```python
from build123d import *

# Parameters (mm, degrees)
ESQUISSE1_W                  = 150
ESQUISSE1_H                  = 150
BOSS_EXTRU_1_DEPTH           = 3
ESQUISSE3_W                  = 130
ESQUISSE3_H                  = 10
ENL_V_MAT_EXTRU_1_DEPTH      = 3
ENL_V_MAT_EXTRU_2_DEPTH      = 153
ENL_V_MAT_EXTRU_2_DEPTH_BACK = 200
ESQUISSE4_R                  = 0.75
CONG_1_R                     = 1
BOSS_EXTRU_5_DEPTH           = 3
BOSS_EXTRU_6_DEPTH           = 3
CONG_4_R                     = 20


with BuildPart() as part:
    # Esquisse1 → Boss.-Extru.1 (new body)
    with BuildSketch(Plane.XY):
        with Locations((75, 75)):
            Rectangle(ESQUISSE1_W, ESQUISSE1_H)
    extrude(amount=BOSS_EXTRU_1_DEPTH)

    # Esquisse3 → Enlèv. mat.-Extru.1 (cut)
    with BuildSketch(Plane.XY.offset(3)):
        with Locations((75, 145)):
            Rectangle(ESQUISSE3_W, ESQUISSE3_H)
    extrude(amount=-ENL_V_MAT_EXTRU_1_DEPTH, mode=Mode.SUBTRACT)

    # Esquisse4 → Enlèv. mat.-Extru.2 (cut, two sides: drawn at the far end of the back side and taken through both)
    with BuildSketch(Plane(origin=(10, 0, 0), x_dir=(0, 0, -1), z_dir=(1, 0, 0)).offset(-ENL_V_MAT_EXTRU_2_DEPTH_BACK)):
        with Locations(Location((-1.5, 148, 0), (0, 0, 270))):
            Circle(ESQUISSE4_R)
    extrude(amount=ENL_V_MAT_EXTRU_2_DEPTH + ENL_V_MAT_EXTRU_2_DEPTH_BACK, mode=Mode.SUBTRACT)

    # Congé1
    cong_1_edges = [part.edges().sort_by_distance(p)[0] for p in [
        (145, 150, 3),
        (5, 150, 0),
        (5, 150, 3),
        (145, 150, 0),
    ]]
    fillet(cong_1_edges, radius=CONG_1_R)

    # Esquisse8 → Boss.-Extru.5 (add)
    with BuildSketch(Plane(origin=(150, 0, 0), x_dir=(0, 0, -1), z_dir=(1, 0, 0))):
        Polygon((0, 3), (68.936542711, -9.155372437), (59.757502948, 47.611044498), (0, 53), align=None)
    extrude(amount=-BOSS_EXTRU_5_DEPTH)

    # Esquisse9 → Boss.-Extru.6 (add)
    with BuildSketch(Plane.ZY):
        Polygon((0, 53), (-59.757502948, 47.611044498), (-68.936542711, -9.155372437), (0, 3), align=None)
    extrude(amount=-BOSS_EXTRU_6_DEPTH)

    # Congé4
    cong_4_edges = [part.edges().sort_by_distance(p)[0] for p in [
        (148.5, 47.611044498, -59.757502948),
        (1.5, 47.611044498, -59.757502948),
    ]]
    fillet(cong_4_edges, radius=CONG_4_R)


solid = part.part
```
Input: part model. Units: mm. Frame: model coordinates. A direction names the side the tool comes from. Coordinates: 2 decimals unless noted, no trailing zeros. Order: outer loops, then holes, each group sorted by start corner. A loop starts at its lowest first (then second) coordinate and runs counter-clockwise, first axis right, second up. Notation, with made-up numbers: (-11.5, 21) - (2.5, 21) arc R26 cw to (2.5, 42) - close; hole circle Ø9 at (38, 50). An arc over 180 degrees is marked (long way). Return JSON: item names as keys, results as strings.
Q1. Cut plane A-A (z = -8.5). Return loops of the section in (x, y).
The answers:
{"outline": "(0, 1.5) - (3, 1.5) - (3, 52.23) - (0, 52.23) - close; (147, 1.5) - (150, 1.5) - (150, 52.23) - (147, 52.23) - close"}
Q2. Draft query along X for faces 1 (the flat face through (150, 29, -25)), 2 (the flat face through (1.479, -3.163, -34.951)), 3 (the flat face through (0, 29, -25)), 4 (the flat face through (74, 76, 0)). Return one class per face: +X half, -X half, draft (parallel to the pull), parting line (faces both ways), or undercut.
The answers:
{"face 1": "+X half", "face 2": "draft", "face 3": "-X half", "face 4": "undercut"}
Q3. Cut plane D-D (y = 109). Return loops of the section in (x, z), then the cut area to 3 significant figures.
The answers:
{"outline": "(0, 0) - (150, 0) - (150, 3) - (0, 3) - close", "area": "450 mm2"}
Q4. Cut plane B-B (z = -19.5). Return loops of the section in (x, y).
The answers:
{"outline": "(0, -0.44) - (3, -0.44) - (3, 51.24) - (0, 51.24) - close; (147, -0.44) - (150, -0.44) - (150, 51.24) - (147, 51.24) - close"}
Q5. Ray query, probe 1 along X at (y, z) = (13.5, -14.5); probe 2 along Z at (x, y) = (143.5, 148); probe 3 along Z at (x, y) = (65.5, 85). Return the intervals inside material, ascending.
The answers:
{"probe 1": "x = 0 to 3, 147 to 150", "probe 2": "z = 0 to 0.75, 2.25 to 3", "probe 3": "z = 0 to 3"}
Q6. Access query for faces 5 (the flat face through (147, 22, -34)), 6 (the flat face through (148.521, -2.993, -33.986)), 7 (the flat face through (148.521, 50.975, -22.455)). Directions: +Z, -Z, +X, -X, +Y, -Y. A direction counts if a zero-diameter tool reaches every point of the face in a straight line with its end or side. Return the directions, or none.
The answers:
{"face 5": "-Z, +Y, -Y", "face 6": "+X, -X, -Y", "face 7": "-Z, +X, -X, +Y"}
Q7. First-contact query: pin 1 (3.5 mm diameter, centred on x = 50, z = 2, fed in from +Y); pin 2 (10 mm diameter, centred on x = 111.5, y = 93, fed in from -Z); pin 3 (2.5 mm diameter, centred on x = 92, z = 2, fed in from -Y). Flat tips, straight axial feed; report the tip coordinate or a pass-through.
The answers:
{"pin 1": "stops at y = 140", "pin 2": "stops at z = 0", "pin 3": "stops at y = 0"}
Q8. Cut plane C-C (x = 70.5). Return loops of the section in (y, z).
The answers:
{"outline": "(0, 0) - (140, 0) - (140, 3) - (0, 3) - close"}
